Part model, mm, in its own coordinate system. A direction names the side the tool comes from. Give positions to 0.01 mm unless a question says otherwise; leave off trailing zeros. Write each loop counter-clockwise with the first axis right and the second up, starting at its lowest first coordinate (ties: lowest second). Pieces come first, ordered by that corner, then holes. Notation, with made-up numbers: (-6.75, -11) - (41.25, -11) arc R29 ccw to (41.25, 18) - close; hole circle Ø1 at (35, 56.5). An arc over 180 degrees is marked (long way). Answer in a Markdown table with one row per item. Add a question column.
1. Band-saw the part on B-B on y = 12.5. Write the cut outline in (x, z).
2. Pull direction Z, two halves, no side cores. Call faces 3 (the flat face through (0, 1, 28)), 4 (the flat face through (-8, 7.8, 9.3)), 5 (the flat face through (-1, 0, -1)): released by +Z, released by -Z, zero draft, split by the parting line, or undercut.
3. Band-saw the part on A-A on x = 0.5. Write the cut outline in (y, z), plus the area to 3 significant figures.
4. Which spindle directions (+Z, -Z, +X, -X, +Y, -Y) get a long thin tool onto all of the face, cutting with end or side? Do faces 1 (the flat face through (6.1, 9, -5)), 2 (the flat face through (-7, 14, -5)). Say none if no direction does.
5. Drop flat-ended pins along their axis: pin 1 Ø2.5 at (x, z) = (-28.5, -1) entering from +Y; pin 2 Ø10 at (x, z) = (-19.5, -20) entering from +Y; pin 3 Ø12 at (x, z) = (-1.5, 25) entering from -Y; pin 4 Ø2 at (x, y) = (1.5, 7.5) entering from +Z. Give the stop position or say it passes through.
6. Probe line 1 along Z through (x, y) = (-23.5, 3); line 2 along Y through (x, z) = (-33, -26); line 3 along X through (y, z) = (4.5, -7.5). List the from-to ranges inside material, lowest first.
7. Band-saw the part on D-D on y = 7.75. Write the cut outline in (x, z), plus the area to 3 significant figures.
```python
from build123d import *

# Parameters (mm, degrees)
BOSS_EXTRUDE1_DEPTH = 4
CUT_EXTRUDE1_DEPTH  = 3
SKETCH3_W           = 26.2
SKETCH3_H           = 36.6
SKETCH3_W_2         = 12.2
SKETCH3_H_2         = 22.6
BOSS_EXTRUDE8_DEPTH = 10
CHAMFER3_SIZE2      = 4.5
CHAMFER3_SIZE       = 10
CHAMFER4_SIZE2      = 10
CHAMFER4_SIZE       = 4.5
CHAMFER5_SIZE       = 10
CHAMFER6_SIZE       = 10
SKETCH4_W           = 6
SKETCH4_H           = 7
CUT_EXTRUDE2_DEPTH  = 69.48999168


# Some blends are built 0.0001 mm under size
with BuildPart() as part:
    # Sketch1 → Boss-Extrude1 (new body)
    with BuildSketch(Plane(origin=(0, 0, 0), x_dir=(1, 0, 0), z_dir=(0, 1, 0))):
        with BuildLine():
            Line((32.908965344, 34), (-32.908965344, 34))
            ThreePointArc((-32.908965344, 34), (-45.899346401, 26.5), (-45.899346401, 11.5))
            Line((-45.899346401, 11.5), (-12.990381057, -45.5))
            ThreePointArc((-12.990381057, -45.5), (0, -53), (12.990381057, -45.5))
            Line((12.990381057, -45.5), (45.899346401, 11.5))
            ThreePointArc((45.899346401, 11.5), (45.899346401, 26.5), (32.908965344, 34))
        make_face()
    extrude(amount=BOSS_EXTRUDE1_DEPTH)

    # Sketch2 → Cut-Extrude1 (cut)
    with BuildSketch(Plane(origin=(0, 4, 0), x_dir=(1, 0, 0), z_dir=(0, 1, 0))):
        with BuildLine():
            Line((4.688500797, 26.589809331), (5.20944533, 29.54423259))
            ThreePointArc((5.20944533, 29.54423259), (0, 30), (-5.20944533, 29.54423259))
            Line((-5.20944533, 29.54423259), (-4.688500797, 26.589809331))
            ThreePointArc((-4.688500797, 26.589809331), (0, 27), (4.688500797, 26.589809331))
        make_face()
        with BuildLine():
            Line((15.486563781, 22.117105196), (17.207293091, 24.574561329))
            ThreePointArc((17.207293091, 24.574561329), (21.213203436, 21.213203436), (24.574561329, 17.207293091))
            Line((24.574561329, 17.207293091), (22.117105196, 15.486563781))
            ThreePointArc((22.117105196, 15.486563781), (19.091883092, 19.091883092), (15.486563781, 22.117105196))
        make_face()
        with BuildLine():
            Line((26.589809331, 4.688500797), (29.54423259, 5.20944533))
            ThreePointArc((29.54423259, 5.20944533), (30, 0), (29.54423259, -5.20944533))
            Line((29.54423259, -5.20944533), (26.589809331, -4.688500797))
            ThreePointArc((26.589809331, -4.688500797), (27, 0), (26.589809331, 4.688500797))
        make_face()
        with BuildLine():
            Line((22.117105196, -15.486563781), (24.574561329, -17.207293091))
            ThreePointArc((24.574561329, -17.207293091), (21.213203436, -21.213203436), (17.207293091, -24.574561329))
            Line((17.207293091, -24.574561329), (15.486563781, -22.117105196))
            ThreePointArc((15.486563781, -22.117105196), (19.091883092, -19.091883092), (22.117105196, -15.486563781))
        make_face()
        with BuildLine():
            Line((4.688500797, -26.589809331), (5.20944533, -29.54423259))
            ThreePointArc((5.20944533, -29.54423259), (0, -30), (-5.20944533, -29.54423259))
            Line((-5.20944533, -29.54423259), (-4.688500797, -26.589809331))
            ThreePointArc((-4.688500797, -26.589809331), (0, -27), (4.688500797, -26.589809331))
        make_face()
        with BuildLine():
            Line((-15.486563781, -22.117105196), (-17.207293091, -24.574561329))
            ThreePointArc((-17.207293091, -24.574561329), (-21.213203436, -21.213203436), (-24.574561329, -17.207293091))
            Line((-24.574561329, -17.207293091), (-22.117105196, -15.486563781))
            ThreePointArc((-22.117105196, -15.486563781), (-19.091883092, -19.091883092), (-15.486563781, -22.117105196))
        make_face()
        with BuildLine():
            Line((-26.589809331, -4.688500797), (-29.54423259, -5.20944533))
            ThreePointArc((-29.54423259, -5.20944533), (-30, 0), (-29.54423259, 5.20944533))
            Line((-29.54423259, 5.20944533), (-26.589809331, 4.688500797))
            ThreePointArc((-26.589809331, 4.688500797), (-27, 0), (-26.589809331, -4.688500797))
        make_face()
        with BuildLine():
            Line((-22.117105196, 15.486563781), (-24.574561329, 17.207293091))
            ThreePointArc((-24.574561329, 17.207293091), (-21.213203436, 21.213203436), (-17.207293091, 24.574561329))
            Line((-17.207293091, 24.574561329), (-15.486563781, 22.117105196))
            ThreePointArc((-15.486563781, 22.117105196), (-19.091883092, 19.091883092), (-22.117105196, 15.486563781))
        make_face()
    extrude(amount=-CUT_EXTRUDE1_DEPTH, mode=Mode.SUBTRACT)

    # Sketch3 → Boss-Extrude8 (add)
    with BuildSketch(Plane(origin=(0, 4, 0), x_dir=(1, 0, 0), z_dir=(0, 1, 0))):
        with Locations((0, 5.2)):
            Rectangle(SKETCH3_W, SKETCH3_H)
        with Locations((0, 5.2)):
            Rectangle(SKETCH3_W_2, SKETCH3_H_2, mode=Mode.SUBTRACT)
    extrude(amount=BOSS_EXTRUDE8_DEPTH)

    # Chamfer3
    chamfer3_edges = [part.edges().sort_by_distance(p)[0] for p in [
        (-13.1, 14, -5.2),
    ]]
    chamfer3_side = [part.faces().sort_by_distance(p)[0] for p in [
        (-13.1, 13.91, -5.2),
    ]]
    chamfer(chamfer3_edges, length=CHAMFER3_SIZE - 0.0001, length2=CHAMFER3_SIZE2 - 0.0001, reference=chamfer3_side[0])  # a hair under: the kernel refuses the full size

    # Chamfer4
    chamfer4_edges = [part.edges().sort_by_distance(p)[0] for p in [
        (13.1, 14, -5.2),
    ]]
    chamfer4_side = [part.faces().sort_by_distance(p)[0] for p in [
        (13.01, 14, -5.2),
    ]]
    chamfer(chamfer4_edges, length=CHAMFER4_SIZE - 0.0001, length2=CHAMFER4_SIZE2 - 0.0001, reference=chamfer4_side[0])  # a hair under: the kernel refuses the full size

    # Chamfer5
    # the kernel refuses this chamfer: 10 mm, written as the material it takes off along each edge
    with BuildSketch(Plane(origin=(-34.31692988, 14, -23.5), x_dir=(0, 0.027495876610586317, 0.9996219169112968), z_dir=(1, 0, 0))) as chamfer5_piece_1_section:
        Polygon((CHAMFER5_SIZE * 0.999621916911, CHAMFER5_SIZE * 0.0274958766106), (-CHAMFER5_SIZE * 0.0274958766106, CHAMFER5_SIZE * 0.999621916911), (0, 0), align=None)
    chamfer5_piece_1 = extrude(amount=68.633859759, mode=Mode.PRIVATE)
    chamfer5_piece_1 = split(chamfer5_piece_1, bisect_by=Plane(origin=(0, 4, -20.195958457), z_dir=(0, 1, 0)), keep=Keep.TOP, mode=Mode.PRIVATE)
    add(chamfer5_piece_1, mode=Mode.SUBTRACT)

    # Chamfer6
    # the kernel refuses this chamfer: 10 mm, written as the material it takes off along each edge
    with BuildSketch(Plane(origin=(34.31692988, 14, 13.1), x_dir=(0, -0.9996219169112968, 0.027495876610586317), z_dir=(-1, 0, 0))) as chamfer6_piece_1_section:
        Polygon((CHAMFER6_SIZE * 0.999621916911, -CHAMFER6_SIZE * 0.0274958766106), (-CHAMFER6_SIZE * 0.0274958766106, -CHAMFER6_SIZE * 0.999621916911), (0, 0), align=None)
    chamfer6_piece_1 = extrude(amount=68.633859759, mode=Mode.PRIVATE)
    chamfer6_piece_1 = split(chamfer6_piece_1, bisect_by=Plane(origin=(0, 4, 9.795958457), z_dir=(0, 1, 0)), keep=Keep.TOP, mode=Mode.PRIVATE)
    add(chamfer6_piece_1, mode=Mode.SUBTRACT)

    # Sketch4 → Cut-Extrude2 (cut, through all)
    with BuildSketch(Plane(origin=(0, 0, 6.1), x_dir=(-1, 0, 0), z_dir=(0, 0, -1))):
        with Locations((0, 7.5)):
            Rectangle(SKETCH4_W, SKETCH4_H)
    extrude(amount=-CUT_EXTRUDE2_DEPTH, mode=Mode.SUBTRACT)


solid = part.part
```
Values:
| question | item | result |
|---|---|---|
| 1 | outline | (-9.28, -15) - (-6.1, -15) - (-6.1, 4.6) - (-9.28, 4.6) - close; (6.1, -15) - (9.28, -15) - (9.28, 4.6) - (6.1, 4.6) - close |
| 2 | face 3 | undercut |
| 2 | face 4 | released by +Z |
| 2 | face 5 | zero draft |
| 3 | outline | (0, -34) - (4, -34) - (4, -30) - (1, -30) - (1, -27) - (4, -27) - (4, -23.5) - (11, -16.5) - (4, -16.5) - (4, 27) - (1, 27) - (1, 30) - (4, 30) - (4, 52.99) - (0, 52.99) - close |
| 3 | area | 354 mm² |
| 4 | face 1 | +Y |
| 4 | face 2 | +Z, -Z, +X, -X, +Y |
| 5 | pin 1 | stops at y = 1 |
| 5 | pin 2 | stops at y = 4 |
| 5 | pin 3 | stops at y = 0 |
| 5 | pin 4 | stops at z = -16.5 |
| 6 | line 1 | z = -34 to -18.65, -16.45 to 16.45, 18.65 to 27.3 |
| 6 | line 2 | y = 0 to 4 |
| 6 | line 3 | x = -12.88 to -6.1, 6.1 to 12.88 |
| 7 | outline | (-11.41, -19.75) - (11.41, -19.75) - (11.41, 9.35) - (3, 9.35) - (3, 6.1) - (6.1, 6.1) - (6.1, -16.5) - (-6.1, -16.5) - (-6.1, 6.1) - (-3, 6.1) - (-3, 9.35) - (-11.41, 9.35) - close |
| 7 | area | 369 mm² |
